Answer from the drawing. Dimensions are ordinates in mm from the lowest x, y and z of the part. A direction names the side the tool comes from. Give positions to 0.01 mm unless a question says otherwise; leave off trailing zeros. Order: outer loops, then holes, each group sorted by start corner. A loop starts at its lowest first (then second) coordinate and runs counter-clockwise, first axis right, second up. Notation, with made-up numbers: (45, 30) -> (73, 30) arc R12 cw to (73, 42) -> close; hole circle Ø5 at (82.5, 21). An arc over 180 degrees is marked (long way). Answer as CSV lines item,"result". Start each with the question number.
1) Find section C-C (y = 8.5). Determine the outline of the cut face in (x, z), and give its area (3 significant figures).
2) Find section A-A (z = 9). Determine the outline of the cut face in (x, y), and give its area (3 significant figures).
3) Find section D-D (y = 11.75). Determine the outline of the cut face in (x, z).
4) For the marked faces 1 and 2, determine the directions among +Z, -Z, +X, -X, +Y, -Y from which every point of the face is accessible in a straight line to the end or side of a thin tool.
5) The mould has two halves that part along Y. Classify the marked faces 3, 4 and 5: +Y half, -Y half, draft (parallel to the pull), parting line (faces both ways), or undercut.
6) Flat-ended cylindrical pins translate along their axes: pin 1 Ø7 at (x, y) = (34, 8) entering from -Z; pin 2 Ø5 at (x, y) = (43.5, 9.5) entering from -Z; pin 3 Ø4 at (x, y) = (37.5, 4.5) entering from -Z. Find the tip coordinate at first contact, or state that the pin passes through.
7) Straight lines are drawn through the part: L1, parallel to Y at x = 43.5, z = 10.25; L2, parallel to Z at x = 3, y = 10. For each, find the intervals that lie inside material, in ascending order. Write a range as from..to.
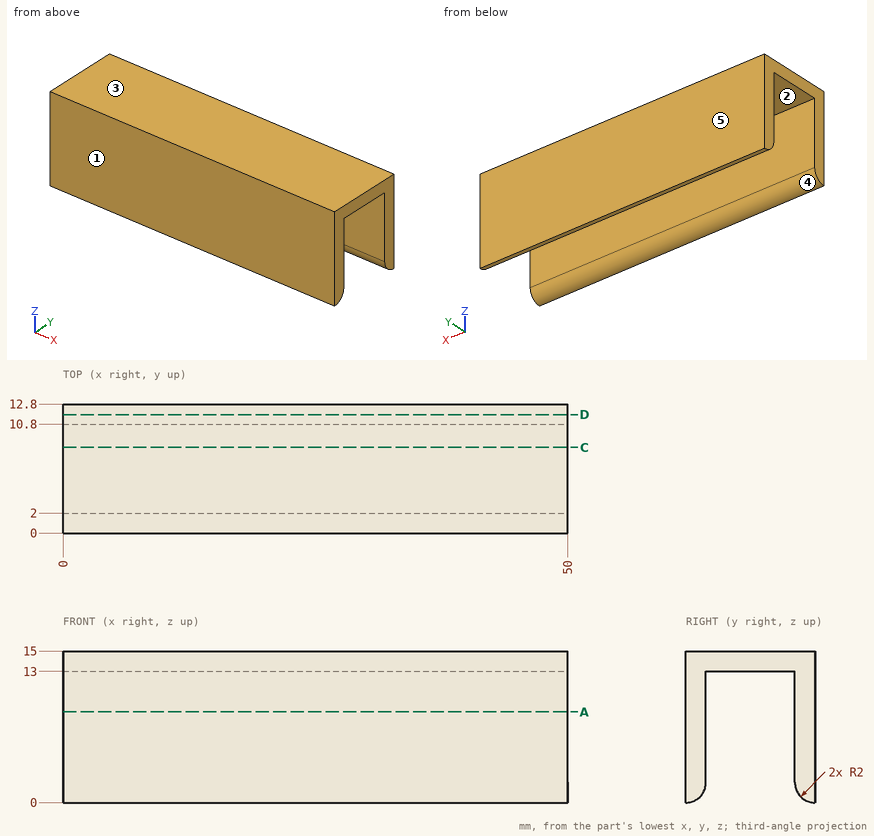
Findings below:
1,outline,"(0, 13) -> (50, 13) -> (50, 15) -> (0, 15) -> close"
1,area,"100 mm²"
2,outline,"(0, 0) -> (50, 0) -> (50, 2) -> (0, 2) -> close; (0, 10.8) -> (50, 10.8) -> (50, 12.8) -> (0, 12.8) -> close"
2,area,"200 mm²"
3,outline,"(0, 0.3) -> (50, 0.3) -> (50, 15) -> (0, 15) -> close"
4,face 1,"+Z, -Z, +X, -X, -Y"
4,face 2,"-Z, +X, -X"
5,face 3,"draft"
5,face 4,"undercut"
5,face 5,"+Y half"
6,pin 1,"z = 0.48"
6,pin 2,"z = 0.17"
6,pin 3,"z = 13"
7,L1,"0..2, 10.8..12.8"
7,L2,"13..15"
